Part model, mm, in its own coordinate system. Coordinates: 2 decimals unless noted, no trailing zeros. Loops run counter-clockwise (first coordinate to the right, second up) from the corner with the lowest first, then second, coordinate; pieces in that order, holes last. Notation, with made-up numbers: M -17,53.25 L 31,53.25 A24 ccw 31,72.25 Z; hole C 50,72.25 d2. An arc over 180 degrees is marked long. Use CSV: the item, a comma, the result in double quotes. Start each with the question number.
from build123d import *

# Parameters (mm, degrees)
CROQUIS1_W              = 0.636
CROQUIS1_H              = 0.636
SALIENTE_EXTRUIR1_DEPTH = 7.8
CROQUIS2_W              = 0.636
CROQUIS2_H              = 0.636
SALIENTE_EXTRUIR2_DEPTH = 7.3
REDONDEO1_R             = 0.5
CHAFL_N1_SIZE           = 0.2
CHAFL_N2_SIZE           = 0.2


with BuildPart() as part:
    # Croquis1 → Saliente-Extruir1 (new body)
    with BuildSketch(Plane(origin=(0, 0, 0), x_dir=(1, 0, 0), z_dir=(0, 1, 0))):
        with Locations((0.318, -0.318)):
            Rectangle(CROQUIS1_W, CROQUIS1_H)
    extrude(amount=SALIENTE_EXTRUIR1_DEPTH)

    # Croquis2 → Saliente-Extruir2 (add)
    with BuildSketch(Plane.XY.offset(0.636)):
        with Locations((0.318, 7.482)):
            Rectangle(CROQUIS2_W, CROQUIS2_H)
    extrude(amount=SALIENTE_EXTRUIR2_DEPTH)

    # Redondeo1
    redondeo1_edges = [part.edges().sort_by_distance(p)[0] for p in [
        (0.318, 7.164, 0.636),
        (0.318, 7.8, 0),
    ]]
    fillet(redondeo1_edges, radius=REDONDEO1_R)

    # Chaflán1
    chafl_n1_edges = [part.edges().sort_by_distance(p)[0] for p in [
        (0.636, 7.482, 7.936),
        (0.318, 7.8, 7.936),
        (0, 7.482, 7.936),
        (0.318, 7.164, 7.936),
    ]]
    chamfer(chafl_n1_edges, length=CHAFL_N1_SIZE)

    # Chaflán2
    chafl_n2_edges = [part.edges().sort_by_distance(p)[0] for p in [
        (0.318, 0, 0),
        (0.636, 0, 0.318),
        (0.318, 0, 0.636),
        (0, 0, 0.318),
    ]]
    chamfer(chafl_n2_edges, length=CHAFL_N2_SIZE)


solid = part.part
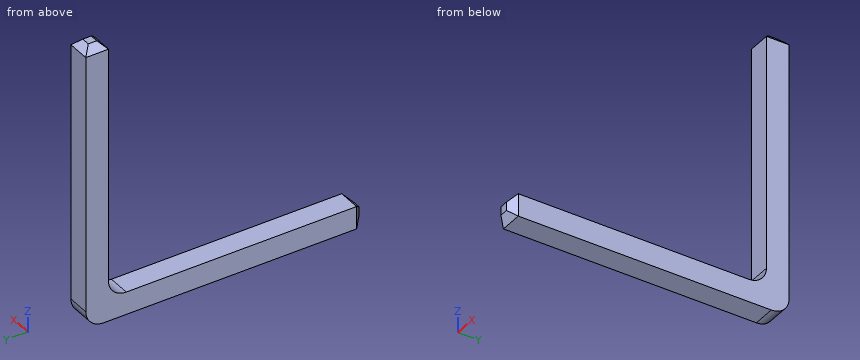
1. Slice it at C-C, the plane z = 7. List the corners of the cut face in (x, y), and give its area (3 significant figures).
2. Slice it at B-B, the plane y = 3.25. List the corners of the cut face in (x, z).
3. Slice it at A-A, the plane x = 0.3. List the corners of the cut face in (y, z), and give its area (3 significant figures).
4. Wall check: probe 1 along Z at (x, y) = (0.3, 1.5); probe 2 along Y at (x, z) = (0.15, 3); probe 3 along Z at (x, y) = (0.05, 7). Give the ranges that are in metal, low to high.
Found:
1,outline,"M 0,7.16 L 0.64,7.16 L 0.64,7.8 L 0,7.8 Z"
1,area,"0.404 mm^2"
2,outline,"M 0,0 L 0.64,0 L 0.64,0.64 L 0,0.64 Z"
3,outline,"M 0,0.2 L 0.2,0 L 7.3,0 A0.5 ccw 7.8,0.5 L 7.8,7.74 L 7.6,7.94 L 7.36,7.94 L 7.16,7.74 L 7.16,1.14 A0.5 cw 6.66,0.64 L 0.2,0.64 L 0,0.44 Z"
3,area,"9.52 mm^2"
4,probe 1,"0 to 0.64"
4,probe 2,"7.16 to 7.8"
4,probe 3,"0 to 0.77"
